```python
from build123d import *

# Parameters (mm, degrees)
SKETCH1_W           = 9.525
SKETCH1_H           = 31.75
BOSS_EXTRUDE1_DEPTH = 0.3175
SKETCH5_W           = 0.508
SKETCH5_H           = 7.62
SKETCH6_R           = 1.6383
CUT_EXTRUDE1_DEPTH  = 12.7


with BuildPart() as part:
    # Sketch1 → Boss-Extrude1 (new, symmetric)
    with BuildSketch(Plane(origin=(0, 0, 0), x_dir=(1, 0, 0), z_dir=(0, 1, 0))):
        Rectangle(SKETCH1_W, SKETCH1_H)
    extrude(amount=BOSS_EXTRUDE1_DEPTH, both=True)

    # Sketch5 → Revolve3 (revolve)
    with BuildSketch(Plane(origin=(0, 0.3175, 0), x_dir=(1, 0, 0), z_dir=(0, 1, 0))):
        with Locations((-4.5085, 4.445)):
            Rectangle(SKETCH5_W, SKETCH5_H)
    revolve3 = revolve(axis=Axis((-6.0325, 0.3175, -15.875), (0, 0, 1)))

    # Mirror2: Revolve3 across plane
    add(revolve3.mirror(Plane.XY))

    # Sketch6 → Cut-Extrude1 (cut)
    with BuildSketch(Plane(origin=(0, 0.3175, 0), x_dir=(1, 0, 0), z_dir=(0, 1, 0))):
        with Locations(Location((0, 0, 0), (0, 0, 270))):
            Circle(SKETCH6_R)
    extrude(amount=-CUT_EXTRUDE1_DEPTH, mode=Mode.SUBTRACT)


solid = part.part
```
Could you check a few things on this model? Use its own coordinates, in mm. Give positions to 0.01 mm unless a question says otherwise; leave off trailing zeros. Loops run counter-clockwise (first coordinate to the right, second up) from the corner with the lowest first, then second, coordinate; pieces in that order, holes last. Notation, with made-up numbers: (49.25, 82.5) - (84.25, 82.5) arc R25 ccw to (84.25, 107.5) - close; hole circle Ø5 at (43.25, 31). An arc over 180 degrees is marked (long way). Answer in a Markdown table with one row per item. Add a question column.
Q1. If we section it at D-D (z = 13): List the corners of the cut face in (x, y) for me, plus the area to 3 significant figures.
Q2. If we section it at A-A (z = 0): List the corners of the cut face in (x, y) for me.
Q3. For pin 1 (1.5 mm diameter, centred on x = -3.5, z = -10, fed in from -Y); pin 2 (1.1 mm diameter, centred on x = -7, y = 1, fed in from -Z) (3 decimals); pin 3 (0.5 mm diameter, centred on y = 0, z = 0, fed in from -X), each with a flat end and sliding along its axis, tell me the tip position at first contact or that it passes through.
Q4. If we section it at C-C (x = 4): List the corners of the cut face in (y, z) for me (1 decimal), plus the area to 3 significant figures.
Q5. We'd pull the mould along Y, two halves only. Please class faces 1 (the face through (2, -0.318, 0)), 2 (the face through (-7.766, 0.713, 4.498)), 3 (the face through (-4.86, -0.17, 4.5)): +Y half, -Y half, draft (parallel to the pull), parting line (faces both ways), or undercut.
Q6. If we section it at B-B (x = 0): List the corners of the cut face in (y, z) for me (1 decimal).
Q7. Please list where these lines run through material, in increasing order: L1, parallel to Z at x = -5.75, y = -1.2 (3 decimals); L2, parallel to X at y = 0.2, z = 0; L3, parallel to Y at x = -1, z = 3.5. Write a range as from..to.
The answers:
| question | item | result |
|---|---|---|
| 1 | outline | (-4.76, -0.32) - (4.76, -0.32) - (4.76, 0.32) - (-4.76, 0.32) - close |
| 1 | area | 6.05 mm^2 |
| 2 | outline | (-4.76, -0.32) - (-1.64, -0.32) - (-1.64, 0.32) - (-4.76, 0.32) - close; (1.64, -0.32) - (4.76, -0.32) - (4.76, 0.32) - (1.64, 0.32) - close |
| 3 | pin 1 | stops at y = -0.32 |
| 3 | pin 2 | stops at z = -8.255 |
| 3 | pin 3 | stops at x = -4.76 |
| 4 | outline | (-0.3, -15.9) - (0.3, -15.9) - (0.3, 15.9) - (-0.3, 15.9) - close |
| 4 | area | 20.2 mm^2 |
| 5 | face 1 | -Y half |
| 5 | face 2 | parting line |
| 5 | face 3 | undercut |
| 6 | outline | (-0.3, -15.9) - (0.3, -15.9) - (0.3, -1.6) - (-0.3, -1.6) - close; (-0.3, 1.6) - (0.3, 1.6) - (0.3, 15.9) - (-0.3, 15.9) - close |
| 7 | L1 | z = -8.255..-0.635, 0.635..8.255 |
| 7 | L2 | x = -4.76..-1.64, 1.64..4.76 |
| 7 | L3 | y = -0.32..0.32 |
